from build123d import *

# Parameters (mm, degrees)
SKETCH_1_W          = 5
SKETCH_1_H          = 2.6
SKETCH_1_W_2        = 23
SKETCH_1_H_2        = 22.75
EXTRUDE_1_DEPTH     = 12.5
SKETCH_2_R          = 5.65
EXTRUDE_2_DEPTH     = 4
SKETCH_3_R          = 2.5
EXTRUDE_3_DEPTH     = 3
SKETCH_4_R          = 0.9
CUT_EXTRUDE_1_DEPTH = 6.5
SKETCH_5_R          = 2.95
EXTRUDE_4_DEPTH     = 4
CUT_EXTRUDE_2_REACH = 20.75
SKETCH_6_R          = 1.25
SKETCH_7_W          = 1.2
SKETCH_7_H          = 3.6
EXTRUDE_5_DEPTH     = 3


with BuildPart() as part:
    # Эскиз1 → Бобышка-Вытянуть1 (new body)
    with BuildSketch(Plane(origin=(0, 0, 0), x_dir=(1, 0, 0), z_dir=(0, 1, 0))):
        with Locations((-2.5, 17.45)):
            Rectangle(SKETCH_1_W, SKETCH_1_H)
        with Locations((11.5, 11.375)):
            Rectangle(SKETCH_1_W_2, SKETCH_1_H_2)
        with Locations((25.5, 17.45)):
            Rectangle(SKETCH_1_W, SKETCH_1_H)
    extrude(amount=EXTRUDE_1_DEPTH)

    # Эскиз2 → Бобышка-Вытянуть2 (add)
    with BuildSketch(Plane(origin=(0, 0, -22.75), x_dir=(-1, 0, 0), z_dir=(0, 0, -1))):
        with Locations((-17.35, 6.25)):
            Circle(SKETCH_2_R)
    extrude(amount=EXTRUDE_2_DEPTH)

    # Эскиз3 → Бобышка-Вытянуть3 (add)
    with BuildSketch(Plane(origin=(0, 0, -26.75), x_dir=(-1, 0, 0), z_dir=(0, 0, -1))):
        with Locations((-17.35, 6.25)):
            Circle(SKETCH_3_R)
    extrude(amount=EXTRUDE_3_DEPTH)

    # Эскиз4 → Вырез-Вытянуть1 (cut)
    with BuildSketch(Plane(origin=(0, 0, -29.75), x_dir=(-1, 0, 0), z_dir=(0, 0, -1))):
        with Locations((-17.35, 6.25)):
            Circle(SKETCH_4_R)
    extrude(amount=-CUT_EXTRUDE_1_DEPTH, mode=Mode.SUBTRACT)

    # Эскиз5 → Бобышка-Вытянуть4 (add)
    with BuildSketch(Plane(origin=(0, 0, -22.75), x_dir=(-1, 0, 0), z_dir=(0, 0, -1))):
        with Locations((-11.35, 6.25)):
            Circle(SKETCH_5_R)
    extrude(amount=EXTRUDE_4_DEPTH)

    # Эскиз6 → Вырез-Вытянуть2 (cut, up to next)
    with BuildSketch(Plane(origin=(0, 0, -18.75), x_dir=(-1, 0, 0), z_dir=(0, 0, -1)), mode=Mode.PRIVATE) as cut_extrude_2_sk1:
        with Locations((2.375, 6.25)):
            Circle(SKETCH_6_R)
    cut_extrude_2_tool1 = extrude(cut_extrude_2_sk1.sketch, amount=-CUT_EXTRUDE_2_REACH, mode=Mode.PRIVATE) & part.part
    add(cut_extrude_2_tool1.solids().sort_by_distance((-2.375, 6.25, -18.75))[0], mode=Mode.SUBTRACT)
    # Эскиз6 → Вырез-Вытянуть2 (cut, up to next)
    with BuildSketch(Plane(origin=(0, 0, -18.75), x_dir=(-1, 0, 0), z_dir=(0, 0, -1)), mode=Mode.PRIVATE) as cut_extrude_2_sk2:
        with Locations((-25.375, 6.25)):
            Circle(SKETCH_6_R)
    cut_extrude_2_tool2 = extrude(cut_extrude_2_sk2.sketch, amount=-CUT_EXTRUDE_2_REACH, mode=Mode.PRIVATE) & part.part
    add(cut_extrude_2_tool2.solids().sort_by_distance((25.375, 6.25, -18.75))[0], mode=Mode.SUBTRACT)

    # Эскиз7 → Бобышка-Вытянуть5 (add)
    with BuildSketch(Plane(origin=(23, 0, 0), x_dir=(0, 0, -1), z_dir=(1, 0, 0))):
        with Locations((4.6, 6.25)):
            Rectangle(SKETCH_7_W, SKETCH_7_H)
    extrude(amount=EXTRUDE_5_DEPTH)


solid = part.part
Model file for the job. Use its own axes, mm. A direction names the side the tool comes from. Coordinates: 2 decimals unless noted, no trailing zeros. Write each loop counter-clockwise with the first axis right and the second up, starting at its lowest first coordinate (ties: lowest second). Pieces come first, ordered by that corner, then holes. Notation, with made-up numbers: (-20.5, 20) -> (1.5, 20) arc R19 cw to (1.5, 52) -> close; hole circle Ø11 at (43.25, -6). An arc over 180 degrees is marked (long way). One line per item, written item: value. Start each with the question number.
1) Pull direction Y, two halves, no side cores. Call faces 1 (the face through (8.4, 6.2, -24.7)), 2 (the face through (17, 6, -23.25)), 3 (the face through (24, 6, -5.2)): +Y half, -Y half, draft (parallel to the pull), parting line (faces both ways), or undercut.
2) Flat gauge pins, fed straight in: pin 1 Ø1 at (y, z) = (7, -10.5) entering from -X; pin 2 Ø4 at (x, y) = (-1.5, 8.5) entering from -Z; pin 3 Ø0.6 at (x, z) = (24.5, -4.5) entering from +Y. Where does each tip first touch, or does it go through?
3) Slice it at D-D on y = 1.25. Write the cut outline in (x, z).
4) Which spindle directions (+Z, -Z, +X, -X, +Y, -Y) get a long thin tool onto all of the face, cutting with end or side? Do faces 4 (the face through (0, 6, -8)), 5 (the face through (24.22, 5.77, -17.47)), 6 (the face through (23, 6, -21)), 7 (the face through (25.5, 4.8, -16.15)). Say none if no direction does.
5) Probe probe 1 along Y at (x, z) = (17.35, -28); probe 2 along X at (y, z) = (6, -10.25); probe 3 along Z at (x, y) = (8.5, 1). List the from-to ranges inside material, lowest first.
6) Slice it at C-C on z = -2. Write the cut outline in (x, y).
7) Slice it at B-B on x = -3. Write the cut outline in (y, z), then the cut area to 3 significant figures.
8) Slice it at A-A on x = 11.35. Write the cut outline in (y, z).
Answers follow:
1. face 1: parting line
1. face 2: undercut
1. face 3: draft
2. pin 1: x = 0
2. pin 2: z = -22.75
2. pin 3: y = 8.05
3. outline: (-5, -18.75) -> (0, -18.75) -> (0, -22.75) -> (14.72, -22.75) -> (14.72, -26.75) -> (19.98, -26.75) -> (19.98, -22.75) -> (23, -22.75) -> (23, -18.75) -> (28, -18.75) -> (28, -16.15) -> (23, -16.15) -> (23, 0) -> (0, 0) -> (0, -16.15) -> (-5, -16.15) -> close
4. face 4: +Z, -X, +Y, -Y
4. face 5: -Z
4. face 6: -Z, +X, +Y, -Y
4. face 7: +X, +Y, -Y
5. probe 1: 3.75 to 5.35, 7.15 to 8.75
5. probe 2: 0 to 23
5. probe 3: -22.75 to 0
6. outline: (0, 0) -> (23, 0) -> (23, 12.5) -> (0, 12.5) -> close
7. outline: (0, -18.75) -> (5.17, -18.75) -> (5.17, -16.15) -> (0, -16.15) -> close; (7.33, -18.75) -> (12.5, -18.75) -> (12.5, -16.15) -> (7.33, -16.15) -> close
7. area: 26.9 mm2
8. outline: (0, -22.75) -> (3.3, -22.75) -> (3.3, -26.75) -> (9.2, -26.75) -> (9.2, -22.75) -> (12.5, -22.75) -> (12.5, 0) -> (0, 0) -> close
